```python
from build123d import *

# Parameters (mm, degrees)
BOSS_EXTRU_1_DEPTH      = 60
ESQUISSE1_3_R           = 1.6
ESQUISSE1_3_R_2         = 7
BOSS_EXTRU_2_DEPTH      = 3
ENL_V_MAT_EXTRU_2_DEPTH = 50
ESQUISSE2_W             = 8
ESQUISSE2_H             = 8
ESQUISSE2_R             = 2.3
ESQUISSE2_H_2           = 16
ESQUISSE2_W_2           = 12
BOSS_EXTRU_4_DEPTH      = 6


with BuildPart() as part:
    # Esquisse1 → Boss.-Extru.1 (new body)
    with BuildSketch(Plane.XY):
        with BuildLine():
            ThreePointArc((18, 0), (12.727922061, -12.727922061), (0, -18))
            Line((0, -18), (18, -18))
            Line((18, -18), (18, 0))
        make_face()
        with BuildLine():
            ThreePointArc((0, -18), (-12.727922061, -12.727922061), (-18, 0))
            Line((-18, 0), (-18, -18))
            Line((-18, -18), (0, -18))
        make_face()
        with BuildLine():
            Line((-14, 0), (-18, 0))
            ThreePointArc((-18, 0), (-12.727922061, -12.727922061), (0, -18))
            ThreePointArc((0, -18), (12.727922061, -12.727922061), (18, 0))
            Line((18, 0), (14, 0))
            ThreePointArc((14, 0), (0, -14), (-14, 0))
        make_face()
    extrude(amount=-BOSS_EXTRU_1_DEPTH)

    # Esquisse1_3 → Boss.-Extru.2 (add)
    with BuildSketch(Plane.XY):
        with BuildLine():
            Line((-13, 18), (-18, 13))
            Line((-18, 13), (-18, 0))
            Line((-18, 0), (-14, 0))
            ThreePointArc((-14, 0), (0, -14), (14, 0))
            Line((14, 0), (18, 0))
            Line((18, 0), (18, 13))
            Line((18, 13), (13, 18))
            Line((13, 18), (-13, 18))
        make_face()
        with Locations((0, 10)):
            Circle(ESQUISSE1_3_R, mode=Mode.SUBTRACT)
        with Locations((0, -10)):
            Circle(ESQUISSE1_3_R, mode=Mode.SUBTRACT)
        with Locations((-10, 0)):
            Circle(ESQUISSE1_3_R, mode=Mode.SUBTRACT)
        Circle(ESQUISSE1_3_R_2, mode=Mode.SUBTRACT)
        with Locations((10, 0)):
            Circle(ESQUISSE1_3_R, mode=Mode.SUBTRACT)
    extrude(amount=-BOSS_EXTRU_2_DEPTH)

    # Esquisse3 → Enl_v. mat.-Extru.2 (cut)
    with BuildSketch(Plane.ZY.offset(18)):
        Polygon((-30, 0), (-20, 0), (-20, -13), (-40, -13), (-40, 0), align=None)
    extrude(amount=-ENL_V_MAT_EXTRU_2_DEPTH, mode=Mode.SUBTRACT)

    # Esquisse2 → Boss.-Extru.4 (add)
    # profile 1 of 3: a face of its own
    with BuildSketch(Plane.XZ.offset(18)):
        with Locations((22, -56)):
            Rectangle(ESQUISSE2_W, ESQUISSE2_H)
        with Locations(Location((22, -56, 0), (0, 0, 270))):
            Circle(ESQUISSE2_R, mode=Mode.SUBTRACT)
    # profile 2 of 3: a face of its own
    with BuildSketch(Plane.XZ.offset(18)):
        with Locations((22, -8)):
            Rectangle(ESQUISSE2_W, ESQUISSE2_H_2)
        with Locations(Location((22, -12, 0), (0, 0, 270))):
            Circle(ESQUISSE2_R, mode=Mode.SUBTRACT)
        with Locations(Location((22, -4, 0), (0, 0, 270))):
            Circle(ESQUISSE2_R, mode=Mode.SUBTRACT)
    # profile 3 of 3: a face of its own
    with BuildSketch(Plane.XZ.offset(18)):
        with Locations((-24, -56)):
            Rectangle(ESQUISSE2_W_2, ESQUISSE2_H)
        with Locations(Location((-26, -56, 0), (0, 0, 270))):
            Circle(ESQUISSE2_R, mode=Mode.SUBTRACT)
    extrude(amount=-BOSS_EXTRU_4_DEPTH)


solid = part.part
```
Geometry check sheet. Reference: the model listing, model coordinates, mm. A direction names the side the tool comes from. Coordinates: 2 decimals unless noted, no trailing zeros. Order: outer loops, then holes, each group sorted by start corner. A loop starts at its lowest first (then second) coordinate and runs counter-clockwise, first axis right, second up. Notation, with made-up numbers: (-6, 66) - (46, 66) arc R19 ccw to (46, 74) - close; hole circle Ø8 at (75, 26.5). An arc over 180 degrees is marked (long way). Answer in a Markdown table with one row per item. Add a question column.
1. Section check A-A (y = 10). Enter the section's corners in (x, z).
2. Material ranges on L1, parallel to Y at x = 0, z = -2.1; L2, parallel to Z at x = 21, y = -13; L3, parallel to Y at x = -17.5, z = -44.5, recorded low to high. Write a range as [from, to].
3. Gauge pin test, flat ends, axial feed: pin 1 Ø12 at (y, z) = (-11.5, -41.5) entering from +X; pin 2 Ø4 at (x, z) = (-27, -56) entering from +Y; pin 3 Ø2 at (x, y) = (-6, 9) entering from -Z. Record the tip position at first contact, or that the pin passes through.
4. Section check B-B (z = -56). Enter the section's corners in (x, y).
5. Section check C-C (x = 22). Enter the section's corners in (y, z).
6. Section check D-D (x = 0). Enter the section's corners in (y, z).
7. Draft check along X on faces 5 (the face through (20.6, -15.042, -10.175)), 6 (the face through (24, -12, -58)), 7 (the face through (16, 15, -1)). Enter one of: +X half, -X half, draft (parallel to the pull), parting line (faces both ways), or undercut.
8. Access from +Z, -Z, +X, -X, +Y, -Y to the whole of each face (thin tool, end or side, straight path). Record for faces 1 (the face through (14, -8, -20)), 2 (the face through (-23, -12, -56)), 3 (the face through (22, -15, -52)), 4 (the face through (22, -12, -8)).
Data:
| question | item | result |
|---|---|---|
| 1 | outline | (-18, -3) - (-1.6, -3) - (-1.6, 0) - (-18, 0) - close; (1.6, -3) - (18, -3) - (18, 0) - (1.6, 0) - close |
| 2 | L1 | y = [-18, -11.6], [-8.4, -7], [7, 8.4], [11.6, 18] |
| 2 | L2 | z = [-60, -58.07], [-53.93, -52], [-16, -14.07], [-9.93, -6.07], [-1.93, 0] |
| 2 | L3 | y = [-18, 0] |
| 3 | pin 1 | stops at x = 18 |
| 3 | pin 2 | stops at y = -12 |
| 3 | pin 3 | stops at z = -3 |
| 4 | outline | (-30, -18) - (-28.3, -18) - (-28.3, -12) - (-30, -12) - close; (-23.7, -18) - (19.7, -18) - (19.7, -12) - (18, -12) - (18, 0) - (14, 0) arc R14 cw to (-14, 0) - (-18, 0) - (-18, -12) - (-23.7, -12) - close; (24.3, -18) - (26, -18) - (26, -12) - (24.3, -12) - close |
| 5 | outline | (-18, -60) - (-12, -60) - (-12, -58.3) - (-18, -58.3) - close; (-18, -53.7) - (-12, -53.7) - (-12, -52) - (-18, -52) - close; (-18, -16) - (-12, -16) - (-12, -14.3) - (-18, -14.3) - close; (-18, -9.7) - (-12, -9.7) - (-12, -6.3) - (-18, -6.3) - close; (-18, -1.7) - (-12, -1.7) - (-12, 0) - (-18, 0) - close |
| 6 | outline | (-18, -60) - (-14, -60) - (-14, -3) - (-11.6, -3) - (-11.6, 0) - (-18, 0) - close; (-8.4, -3) - (-7, -3) - (-7, 0) - (-8.4, 0) - close; (7, -3) - (8.4, -3) - (8.4, 0) - (7, 0) - close; (11.6, -3) - (18, -3) - (18, 0) - (11.6, 0) - close |
| 7 | face 5 | undercut |
| 7 | face 6 | draft |
| 7 | face 7 | +X half |
| 8 | face 1 | +X, -X, +Y |
| 8 | face 2 | +Z, -Z, -X, +Y |
| 8 | face 3 | +X, +Y, -Y |
| 8 | face 4 | +Z, -Z, +X, +Y |
